```python
from build123d import *

# Parameters (mm, degrees)
CROQUIS1_W                       = 40
CROQUIS1_H                       = 40
BRIDA_BASE1_DEPTH                = 2
BRIDA_DE_ARISTA1_STRIP_W         = 9.4732
BRIDA_DE_ARISTA1_STRIP_H         = 2
BRIDA_DE_ARISTA1_STRIP_CUT_DEPTH = 40
BRIDA_DE_ARISTA1_DEPTH           = 40
CORTAR_EXTRUIR2_REACH            = 54.383
CROQUIS11_R                      = 8


# Sheet-metal steps are written as plain solids
with BuildPart() as part:
    # Croquis1 → Brida base1 (new body)
    with BuildSketch(Plane.XY):
        Rectangle(CROQUIS1_W, CROQUIS1_H)
    extrude(amount=BRIDA_BASE1_DEPTH)

    # Brida de arista1 strip (across the edge) → Brida de arista1 strip cut (cut)
    with BuildSketch(Plane(origin=(20, -20, 2), x_dir=(-1, 0, 0), z_dir=(0, 1, 0))):
        with Locations((-2, -1)):
            Rectangle(BRIDA_DE_ARISTA1_STRIP_W, BRIDA_DE_ARISTA1_STRIP_H)
    extrude(amount=BRIDA_DE_ARISTA1_STRIP_CUT_DEPTH, mode=Mode.SUBTRACT)

    # Brida de arista1 section (across the edge) → Brida de arista1 (add)
    with BuildSketch(Plane(origin=(20, -20, 2), x_dir=(-1, 0, 0), z_dir=(0, 1, 0))):
        with BuildLine():
            Line((0, 0.7366), (0, 28))
            Line((0, 28), (2, 28))
            Line((2, 28), (2, 0.7366))
            ThreePointArc((2, 0.7366), (2.215745145, 0.215745145), (2.7366, 0))
            Line((2.7366, 0), (2.7366, -2))
            ThreePointArc((2.7366, -2), (0.801531583, -1.198468417), (0, 0.7366))
        make_face()
    extrude(amount=BRIDA_DE_ARISTA1_DEPTH)

    # Croquis11 → Cortar-Extruir2 (cut, up to next)
    with BuildSketch(Plane.ZY.offset(-18), mode=Mode.PRIVATE) as cortar_extruir2_sk1:
        with Locations((12.31, 0)):
            Circle(CROQUIS11_R)
    cortar_extruir2_tool1 = extrude(cortar_extruir2_sk1.sketch, amount=-CORTAR_EXTRUIR2_REACH, mode=Mode.PRIVATE) & part.part
    add(cortar_extruir2_tool1.solids().sort_by_distance((18, 0, 12.31))[0], mode=Mode.SUBTRACT)


solid = part.part
```
For this review, take the finished solid that the model builds, in its own axes (mm). A direction names the side the tool comes from. Round coordinates to 2 decimals unless told otherwise and drop trailing zeros. Write each loop counter-clockwise with the first axis right and the second up, starting at its lowest first coordinate (ties: lowest second). Pieces come first, ordered by that corner, then holes. Notation, with made-up numbers: M 74,-29 L 101,-29 A11 ccw 101,-20 Z; hole C 26.5,-33 d10. An arc over 180 degrees is marked long. One line per item, written item: value. Start each with the question number.
(1) Insertion check: pin 1 (8 mm diameter, centred on x = 7.5, y = -16, fed in from +Z); pin 2 (10 mm diameter, centred on x = 7.5, z = 10.5, fed in from -Y). Each pin has a flat end and moves straight along its axis. Give the tip position at first contact, or say it passes through.
(2) The part is to be moulded in two halves that separate along Y. For faces 3 (the flat face through (-2, 0, 0)), 4 (the flat face through (5.8, -20, 1.7)), 5 (the cylindrical face through (18.99, -3.06, 19.7)), say which applies: released by +Y, released by -Y, zero draft, split by the parting line, or undercut.
(3) We need section C-C (y = -17). Give the boundary of the cut face in (x, z), and give its area (3 significant figures).
(4) We need section A-A (y = 0). Give the boundary of the cut face in (x, z), and give its area (3 significant figures).
(5) Machinability: for faces 1 (the flat face through (-2, 0, 2)), 2 (the cylindrical face through (19.177, -0.28, 0.78)), which of the approach directions +Z, -Z, +X, -X, +Y, -Y give a long, thin tool a straight path to every point of the face, cutting with its end or side? Answer none if there is none.
(6) We need section B-B (z = 12.31). Give the boundary of the cut face in (x, y), and give its area (3 significant figures).
(7) Wall thickness on line 1 (Y direction, x = 19.2, z = 12.31); line 2 (X direction, y = 16, z = 17.25); line 3 (Z direction, x = 11.5, y = 17): over which ranges is each line inside the solid? List them lowest first.
(8) We need section D-D (z = 7.25). Give the boundary of the cut face in (x, y).
Result:
1. pin 1: z = 2
1. pin 2: through
2. face 3: zero draft
2. face 4: released by -Y
2. face 5: undercut
3. outline: M -20,0 L 17.26,0 A2.74 ccw 20,2.74 L 20,30 L 18,30 L 18,2.74 A0.74 cw 17.26,2 L -20,2 Z
3. area: 135 mm²
4. outline: M -20,0 L 17.26,0 A2.74 ccw 20,2.74 L 20,4.31 L 18,4.31 L 18,2.74 A0.74 cw 17.26,2 L -20,2 Z; M 18,20.31 L 20,20.31 L 20,30 L 18,30 Z
4. area: 103 mm²
5. face 1: +Z, -X, +Y, -Y
5. face 2: -Z, +X, +Y, -Y
6. outline: M 18,-20 L 20,-20 L 20,-8 L 18,-8 Z; M 18,8 L 20,8 L 20,20 L 18,20 Z
6. area: 48.0 mm²
7. line 1: -20 to -8, 8 to 20
7. line 2: 18 to 20
7. line 3: 0 to 2
8. outline: M 18,-20 L 20,-20 L 20,-6.2 L 18,-6.2 Z; M 18,6.2 L 20,6.2 L 20,20 L 18,20 Z
